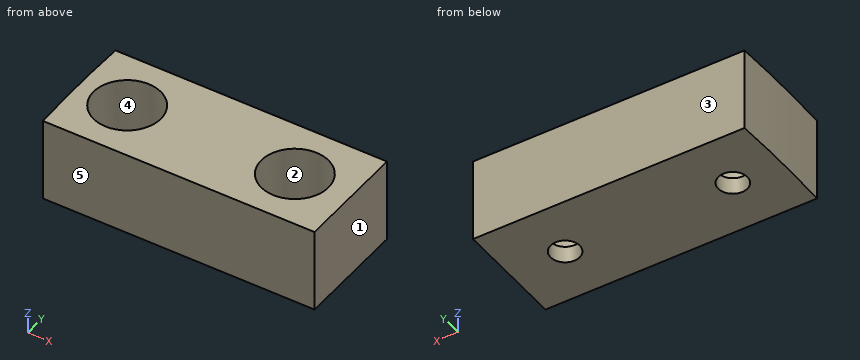
Autodesk Inventor part; units mm, degrees
ref_plane "YZ Plane" through (0, 0, 0) normal (1, 0, 0) x (0, 1, 0)
ref_plane "XZ Plane" through (0, 0, 0) normal (0, 1, 0) x (-1, 0, 0)
ref_plane "XY Plane" through (0, 0, 0) normal (0, 0, 1) x (1, 0, 0)
sketch "Sketch1" plane through (0, 0, 0) normal (0, 0, 1) x (1, 0, 0)
  arc A0 (-243.5713, 10) -> (-243.5713, -10) centre (0, 0) ccw
  line L0 (-195, -10) -> (-195, 10)
  line L1 (-195, 10) -> (-243.5713, 10)
  line L2 (-195, -10) -> (-195, -10)
  line L3 (-195, -10) -> (-243.5713, -10)
  dimension "d19" = 10
  dimension "d20" = 10
  dimension "d21" = 0
extrude "Extrusion1" add sketch "Sketch1" along normal blind 15
sketch "Sketch2" plane through (0, 0, 15) normal (0, 0, 1) x (1, 0, 0)
  circle A0 centre (-205, 0) radius 2.6
  line L0 (-195, -10) -> (-195, 10)
  circle A1 centre (-235, 0) radius 2.6
  point P0 (0, 0)
  dimension "d6" = 5.2
  dimension "d7" = 10
  dimension "d8" = 10
  dimension "d9" = 5.2
  dimension "d10" = 10
  dimension "d11" = 30
hole "Hole1" at (-235, 0, 15) at (-205, 0, 15) direction (0, 0, -1) diameter 5.2 end through all counterbore diameter 12 counterbore depth 12
properties part number "turntable_hit"
Source: CAD feature listing. Evaluate the final solid. Frame: model axes, mm. Face numbers are marked on the shaded views. A direction names the side the tool comes from. Give positions to 0.01 mm unless a question says otherwise; leave off trailing zeros. Order: outer loops, then holes, each group sorted by start corner. A loop starts at its lowest first (then second) coordinate and runs counter-clockwise, first axis right, second up.
(1) Section query B-B (x = -205). Return the cut outline in (y, z).
(2) Material intervals for line 1 along X through (y, z) = (0.5, 9.25); line 2 along Y through (x, z) = (-205, 8); line 3 along Y through (x, z) = (-205, 1.55), sorted ascending.
(3) Section query A-A (y = 0). Return the cut outline in (x, z), plus the area to 3 significant figures.
(4) Section query D-D (x = -230). Return the cut outline in (y, z).
(5) Contact query for flat-ended pins moving along their axis: P1, Ø7, axis at x = -235, y = 0, coming from the +Z side; P2, Ø1, axis at y = -4.5, z = 5.5, coming from the -X side; P3, Ø3, axis at x = -225, y = -7.5, coming from the -Z side. Output: stop coordinate, or through.
(6) Section query C-C (z = 7). Return the cut outline in (x, y).
(7) Pull-direction query (Y, two-part tool) for the marked faces 1, 2 and 3; classes: +Y half, -Y half, draft (parallel to the pull), parting line (faces both ways), or undercut.
(8) Access query for the marked faces 4 and 5. Directions: +Z, -Z, +X, -X, +Y, -Y. A direction counts if a zero-diameter tool reaches every point of the face in a straight line with its end or side. Return the directions, or none.
Outcome:
1. outline: (-10, 0) - (-2.6, 0) - (-2.6, 3) - (-6, 3) - (-6, 15) - (-10, 15) - close; (2.6, 0) - (10, 0) - (10, 15) - (6, 15) - (6, 3) - (2.6, 3) - close
2. line 1: x = -243.78 to -240.98, -229.02 to -210.98, -199.02 to -195
2. line 2: y = -10 to -6, 6 to 10
2. line 3: y = -10 to -2.6, 2.6 to 10
3. outline: (-243.78, 0) - (-237.6, 0) - (-237.6, 3) - (-241, 3) - (-241, 15) - (-243.78, 15) - close; (-232.4, 0) - (-207.6, 0) - (-207.6, 3) - (-211, 3) - (-211, 15) - (-229, 15) - (-229, 3) - (-232.4, 3) - close; (-202.4, 0) - (-195, 0) - (-195, 15) - (-199, 15) - (-199, 3) - (-202.4, 3) - close
3. area: 412 mm2
4. outline: (-10, 0) - (10, 0) - (10, 15) - (3.32, 15) - (3.32, 3) - (-3.32, 3) - (-3.32, 15) - (-10, 15) - close
5. P1: stops at z = 3
5. P2: stops at x = -243.74
5. P3: stops at z = 0
6. outline: (-243.57, -10) - (-195, -10) - (-195, 10) - (-243.57, 10) arc R243.78 ccw to start; hole circle Ø12 at (-235, 0); hole circle Ø12 at (-205, 0)
7. face 1: draft
7. face 2: undercut
7. face 3: +Y half
8. face 4: +Z
8. face 5: +Z, -Z, +X, -X, -Y
